The listing builds one solid part. Answer for the finished solid, in the listing's coordinates (mm). Face numbers are marked on the shaded views. A direction names the side the tool comes from. Round coordinates to 2 decimals unless told otherwise and drop trailing zeros. Write each loop counter-clockwise with the first axis right and the second up, starting at its lowest first coordinate (ties: lowest second). Pieces come first, ordered by that corner, then holes. Notation, with made-up numbers: (56.25, -1) - (75.25, -1) arc R27 ccw to (75.25, 15) - close; hole circle Ø1 at (38, -9.75). An arc over 180 degrees is marked (long way). Answer in a Markdown table with one row per item.
from build123d import *

# Parameters (mm, degrees)
F1_DEPTH = 20
F2_R     = 2
F3_DEPTH = 18.001


with BuildPart() as f1:
    # F0 (on Front) → F1 (new body, symmetric)
    with BuildSketch(Plane.XZ):
        Polygon((-10, 45), (-10, 0), (0, 0), (0, 53), (-18, 53), (-18, 45), align=None)
    extrude(amount=F1_DEPTH, both=True)

    # F2 (on face) → F3 (cut, through all)
    with BuildSketch(Plane.YZ):
        with Locations((-10, 15)):
            Circle(F2_R)
        with Locations((10, 15)):
            Circle(F2_R)
    extrude(amount=-F3_DEPTH, mode=Mode.SUBTRACT)


solid = f1.part
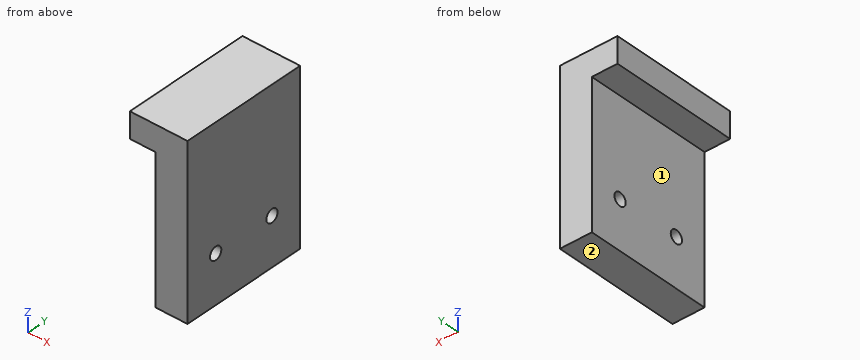
(1) Section A-A (y = -10) is taken. Give the vertices of the cut face in (x, z).
Checked values:
| item | result |
|---|---|
| outline | (-18, 45) - (-10, 45) - (-10, 17) - (0, 17) - (0, 53) - (-18, 53) - close; (-10, 0) - (0, 0) - (0, 13) - (-10, 13) - close |
(2) Section B-B (z = 15) is taken. Give the vertices of the cut face in (x, y), and give its area (3 significant figures).
Checked values:
| item | result |
|---|---|
| outline | (-10, -20) - (0, -20) - (0, -12) - (-10, -12) - close; (-10, -8) - (0, -8) - (0, 8) - (-10, 8) - close; (-10, 12) - (0, 12) - (0, 20) - (-10, 20) - close |
| area | 320 mm2 |
(3) For the marked faces 1 and 2, determine the directions among +Z, -Z, +X, -X, +Y, -Y from which every point of the face is accessible in a straight line to the end or side of a thin tool.
Checked values:
| item | result |
|---|---|
| face 1 | -Z, -X, +Y, -Y |
| face 2 | -Z, +X, -X, +Y, -Y |
(4) Section D-D (z = 5.5) is taken. Give the vertices of the cut face in (x, y).
Checked values:
| item | result |
|---|---|
| outline | (-10, -20) - (0, -20) - (0, 20) - (-10, 20) - close |
(5) Find the intervals of material crossed by line 1 (Z direction, x = -5.5, y = 10); line 2 (X direction, y = -2, z = 29); line 3 (Z direction, x = -17, y = 9.5), in increasing order.
Checked values:
| item | result |
|---|---|
| line 1 | z = 0 to 13, 17 to 53 |
| line 2 | x = -10 to 0 |
| line 3 | z = 45 to 53 |
(6) Section C-C (y = 0) is taken. Give the vertices of the cut face in (x, z).
Checked values:
| item | result |
|---|---|
| outline | (-18, 45) - (-10, 45) - (-10, 0) - (0, 0) - (0, 53) - (-18, 53) - close |
